Check sheet for the modelled part. Datum: model origin and axes. Units: mm. Face numbers are marked on the shaded views. A direction names the side the tool comes from. Coordinates: 2 decimals unless noted, no trailing zeros. Loops run counter-clockwise (first coordinate to the right, second up) from the corner with the lowest first, then second, coordinate; pieces in that order, holes last. Notation, with made-up numbers: (65.25, 82) -> (124.25, 82) arc R11 cw to (124.25, 100) -> close; hole circle Ø5 at (9, 86). An arc over 180 degrees is marked (long way). Use CSV: the item, a comma, the result in double quotes.
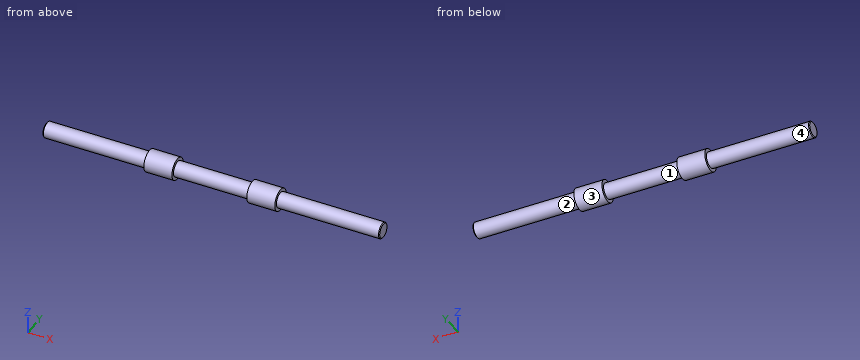
Autodesk Inventor part; units mm, degrees
ref_plane "YZ Plane" through (0, 0, 0) normal (1, 0, 0) x (0, 1, 0)
ref_plane "XZ Plane" through (0, 0, 0) normal (0, 1, 0) x (-1, 0, 0)
ref_plane "XY Plane" through (0, 0, 0) normal (0, 0, 1) x (1, 0, 0)
sketch "草图1" plane through (0, 0, 0) normal (0, 0, 1) x (1, 0, 0)
  line L0 (0, 0) -> (0, 2.5)
  line L1 (0, 2.5) -> (5, 2.5)
  line L2 (5, 2.5) -> (33, 2.5)
  line L3 (33, 2.5) -> (33, 3.5)
  line L4 (33, 3.5) -> (42, 3.5)
  line L5 (42, 3.5) -> (42, 2.5)
  line L6 (42, 2.5) -> (66, 2.5)
  line L7 (66, 2.5) -> (66, 3.5)
  line L8 (66, 3.5) -> (75, 3.5)
  line L9 (75, 3.5) -> (75, 2.5)
  line L10 (75, 2.5) -> (108, 2.5)
  line L11 (108, 2.5) -> (108, 0)
  line L12 (108, 0) -> (0, 0)
  line L13 (-21.6, 0) -> (129.6, 0)
  dimension "d0" = 2.5
  dimension "d1" = 5
  dimension "d2" = 28
  dimension "d3" = 1
  dimension "d4" = 9
  dimension "d5" = 24
  dimension "d6" = 9
  dimension "d7" = 33
revolve "旋转1" add sketch "草图1" angle 360 about axis through (-10, 0, 0) along (1, 0, 0)
thread "螺纹1"
thread "螺纹2"
chamfer "倒角1" distance 0.25 angle 45 2 edges at (108, -2.5, 0) (0, -2.5, 0)
properties part number "刮肉轮轴"
1) Go/stop test with flat-tipped pins: pin 1 Ø3 at (x, y) = (86.5, 1) entering from -Z; pin 2 Ø4 at (x, y) = (44.5, 2) entering from +Z. Record where each tip stops, or that it passes through.
Answer below:
pin 1,"stops at z = -2.5"
pin 2,"stops at z = 2.5"
2) Thickness scan on line 1 along X through (y, z) = (2, 2.5); line 2 along Z through (x, y) = (56, 0.25); line 3 along Y through (x, z) = (20.5, -1.5). Record the ranges inside material, lowest first. Write a range as from..to.
Answer below:
line 1,"x = 33..42, 66..75"
line 2,"z = -2.49..2.49"
line 3,"y = -2..2"
3) Cross-section at A-A on y = 0. Record the boundary of the cut face in (x, z).
Answer below:
outline,"(0, -2.25) -> (0.25, -2.5) -> (33, -2.5) -> (33, -3.5) -> (42, -3.5) -> (42, -2.5) -> (66, -2.5) -> (66, -3.5) -> (75, -3.5) -> (75, -2.5) -> (107.75, -2.5) -> (108, -2.25) -> (108, 2.25) -> (107.75, 2.5) -> (75, 2.5) -> (75, 3.5) -> (66, 3.5) -> (66, 2.5) -> (42, 2.5) -> (42, 3.5) -> (33, 3.5) -> (33, 2.5) -> (0.25, 2.5) -> (0, 2.25) -> close"
4) Draft check along X on the marked faces 1 and 2. Enter one of: released by +X, released by -X, zero draft, split by the parting line, or undercut.
Answer below:
face 1,"undercut"
face 2,"zero draft"
5) Cross-section at C-C on x = 14. Record the boundary of the cut face in (y, z), and give its area (3 significant figures).
Answer below:
outline,"circle Ø5 at (0, 0)"
area,"19.6 mm²"
6) Access from +Z, -Z, +X, -X, +Y, -Y to the whole of each face (thin tool, end or side, straight path). Record for the marked faces 3 and 4.
Answer below:
face 3,"+X, -X"
face 4,"-X"
